Design review of the part built by this model. Coordinates are the model's own, in mm. A direction names the side the tool comes from. Round coordinates to 2 decimals unless told otherwise and drop trailing zeros. Loops run counter-clockwise (first coordinate to the right, second up) from the corner with the lowest first, then second, coordinate; pieces in that order, holes last. Notation, with made-up numbers: (-11, -18) - (8, -18) arc R29 cw to (8, 17) - close; hole circle Ø9 at (43, 26). An arc over 180 degrees is marked (long way). Use one line per item in the form item = value. Start each with the question number.
(1) We need section A-A, the plane y = 1.9. Write out the cut boundary in (x, z).
(2) Machinability: for faces 1 (the flat face through (-15, 3, 0)), 2 (the flat face through (-3, 2, -1.95)), which of the approach directions +Z, -Z, +X, -X, +Y, -Y give a long, thin tool a straight path to every point of the face, cutting with its end or side? Answer none if there is none.
(3) For pin 1 (2 mm diameter, centred on y = 1.5, z = -0.5, fed in from -X), flat-tipped, find the tip position at first contact; note if it passes through.
(4) The part is to be moulded in two halves that separate along Z. For faces 3 (the flat face through (0, 2, -7.5)), 4 (the flat face through (9.45, 2, 0)), 5 (the cylindrical face through (-2.95, 1.09, 1.78)), 6 (the flat face through (0, 2, 7.5)), say which applies: released by +Z, released by -Z, zero draft, split by the parting line, or undercut.
(5) Wall thickness on probe 1 along Z at (x, y) = (-3.25, 2); probe 2 along Z at (x, y) = (-9.5, 0.6); probe 3 along Y at (x, z) = (4, -0.5): over which ranges is each line inside the solid? List them lowest first. Write a range as [from, to].
(6) We need section B-B, the plane x = 8.5. Write out the cut boundary in (y, z), then the cut area to 3 significant figures.
from build123d import *

# Parameters (mm, degrees)
SKETCH_1_W          = 30
SKETCH_1_H          = 15
EXTRUDE_1_DEPTH     = 5
CUT_EXTRUDE_1_DEPTH = 24.45
FILLET_1_R          = 0.2


with BuildPart() as part:
    # 草图1 → 凸台-拉伸1 (new body)
    with BuildSketch(Plane(origin=(0, 0, 0), x_dir=(1, 0, 0), z_dir=(0, 1, 0))):
        Rectangle(SKETCH_1_W, SKETCH_1_H)
    extrude(amount=EXTRUDE_1_DEPTH)

    # 草图2 → 切除-拉伸1 (cut)
    with BuildSketch(Plane.ZY.offset(15)):
        with BuildLine():
            Line((-1.5, 0), (-1.5, 0.677124344))
            ThreePointArc((-1.5, 0.677124344), (-1.780042303, 1.088161527), (-1.95, 1.555590279))
            Line((-1.95, 1.555590279), (-1.95, 2.8))
            Line((-1.95, 2.8), (1.95, 2.8))
            Line((1.95, 2.8), (1.95, 1.555590279))
            ThreePointArc((1.95, 1.555590279), (1.780042303, 1.088161527), (1.5, 0.677124344))
            Line((1.5, 0.677124344), (1.5, 0))
            Line((1.5, 0), (-1.5, 0))
        make_face()
    extrude(amount=-CUT_EXTRUDE_1_DEPTH, mode=Mode.SUBTRACT)

    # 圆角1
    fillet_1_edges = [part.edges().sort_by_distance(p)[0] for p in [
        (15, 5, 0),
        (0, 5, -7.5),
        (-15, 0, 4.5),
        (9.45, 0, 0),
        (-2.775, 0, 1.5),
        (-2.775, 0, -1.5),
        (-15, 5, 0),
        (0, 0, -7.5),
        (15, 0, 0),
        (0, 0, 7.5),
        (-15, 0, -4.5),
        (0, 5, 7.5),
        (-15, 2.5, -7.5),
        (15, 2.5, -7.5),
        (15, 2.5, 7.5),
        (-15, 2.5, 7.5),
    ]]
    fillet(fillet_1_edges, radius=FILLET_1_R)


solid = part.part
Data:
q1.outline = (-15, -7.3) arc R0.2 ccw to (-14.8, -7.5) - (14.8, -7.5) arc R0.2 ccw to (15, -7.3) - (15, 7.3) arc R0.2 ccw to (14.8, 7.5) - (-14.8, 7.5) arc R0.2 ccw to (-15, 7.3) - (-15, 1.95) - (9.45, 1.95) - (9.45, -1.95) - (-15, -1.95) - close
q2.face_1 = +Z, -Z, -X, +Y, -Y
q2.face_2 = -X
q3.pin_1 = 9.45
q4.face_3 = released by -Z
q4.face_4 = undercut
q4.face_5 = undercut
q4.face_6 = released by +Z
q5.probe_1 = [-7.5, -1.95], [1.95, 7.5]
q5.probe_2 = [-7.5, -1.5], [1.5, 7.5]
q5.probe_3 = [2.8, 5]
q6.outline = (0, -7.3) arc R0.2 ccw to (0.2, -7.5) - (4.8, -7.5) arc R0.2 ccw to (5, -7.3) - (5, 7.3) arc R0.2 ccw to (4.8, 7.5) - (0.2, 7.5) arc R0.2 ccw to (0, 7.3) - (0, 1.7) arc R0.2 ccw to (0.2, 1.5) - (0.68, 1.5) arc R2 cw to (1.56, 1.95) - (2.8, 1.95) - (2.8, -1.95) - (1.56, -1.95) arc R2 cw to (0.68, -1.5) - (0.2, -1.5) arc R0.2 ccw to (0, -1.7) - close
q6.area = 65.0 mm^2
